from build123d import *

# Parameters (mm, degrees)
SKETCH2_R         = 4.7625
CIRPATTERN1_COUNT = 2


with BuildPart() as part:
    # Sweep1: sweep along a path in Sketch1
    with BuildLine(Plane(origin=(0, 0, 0), x_dir=(1, 0, 0), z_dir=(0, 1, 0))) as sweep1_path:
        Line((0, 0), (-15.875, 0))
        ThreePointArc((-15.875, 0), (-31.608119304, 17.992683159), (-11.677486704, 31.185013296))
        Line((-11.677486704, 31.185013296), (3.632526592, 26.9875))
    # Sketch2 → Sweep1 (sweep)
    with BuildSketch(Plane(origin=(0, 0, 0), x_dir=(0, 0, -1), z_dir=(1, 0, 0))):
        Circle(SKETCH2_R)
    sweep1 = sweep(path=sweep1_path.line)

    # CirPattern1: Sweep1 ×2 about axis
    cirpattern1_axis = Axis((0, 0, 0), (0, 1, 0))
    for i in range(1, CIRPATTERN1_COUNT):
        add(sweep1.rotate(cirpattern1_axis, i * 360 / CIRPATTERN1_COUNT))


solid = part.part
Geometry check sheet. Reference: the model listing, model coordinates, mm. Give positions to 0.01 mm unless a question says otherwise; leave off trailing zeros. Write each loop counter-clockwise with the first axis right and the second up, starting at its lowest first coordinate (ties: lowest second). Pieces come first, ordered by that corner, then holes.
1) Thickness scan on line 1 (Z direction, x = 22.5, y = 1.5); line 2 (Z direction, x = 12, y = 0.75); line 3 (X direction, y = 0, z = -1). Record the ranges inside material, lowest first.
Values follow:
line 1: z = -3.41 to 6.65, 25.1 to 35.16
line 2: z = -4.7 to 4.7, 26.4 to 36.08
line 3: x = -30.18 to 27.76
2) Cross-section at B-B (x = 4). Count the separate pieces of the cut face and the enclosed holes in it, plus the area to 3 significant figures.
Values follow:
separate pieces: 3
enclosed holes: 0
area: 169 mm2
3) Cross-section at A-A (y = -2). Record the boundary of the cut face in (x, z) (3 decimals).
Values follow:
outline: (-15.875, -4.322) - (15.875, -4.322) arc R20.197 ccw (long way) to (10.535, 35.353) - (-4.775, 31.156) - (-2.49, 22.819) - (12.82, 27.017) arc R11.553 cw (long way) to (15.875, 4.322) - (-15.875, 4.322) arc R20.197 ccw (long way) to (-10.535, -35.353) - (4.775, -31.156) - (2.49, -22.819) - (-12.82, -27.017) arc R11.553 cw (long way) to start
4) Release check for a two-part mould opening along X. For faces 1 (the face through (5.079, 1.824, 24.814)), 2 (the face through (3.615, -0.067, -26.923)), 3 (the face through (-3.615, -0.067, 26.923)) record: released by +X, released by -X, zero draft, split by the parting line, or undercut.
Values follow:
face 1: undercut
face 2: released by +X
face 3: released by -X
5) Go/stop test with flat-tipped pins: pin 1 Ø2 at (y, z) = (-1, 16.5) entering from +X; pin 2 Ø1.5 at (y, z) = (-3, -19) entering from +X; pin 3 Ø1 at (x, y) = (16, -0.5) entering from -Z. Record where each tip stops, or that it passes through.
Values follow:
pin 1: stops at x = 36.51
pin 2: stops at x = -27.07
pin 3: stops at z = -4.76
